Here's how the part is built. I have some questions about the finished solid (model axes, mm). Face numbers are marked on the shaded views. A direction names the side the tool comes from. Give positions to 0.01 mm unless a question says otherwise; leave off trailing zeros. Loops run counter-clockwise (first coordinate to the right, second up) from the corner with the lowest first, then second, coordinate; pieces in that order, holes last. Notation, with made-up numbers: (7.25, 47) - (27.25, 47) arc R25 ccw to (27.25, 85) - close; hole circle Ø1 at (84.25, -5.75). An arc over 180 degrees is marked (long way). Use a Markdown table: item, result.
Solid Edge part; units mm, degrees
sketch "Sketch1" plane through (0, 0, 0) normal (0, 0, 1) x (1, 0, 0)
  circle A0 centre (-61.7143, 32.036) radius 10
extrude "Protrusion1" add sketch "Sketch1" along normal blind 35
sketch "Sketch2" plane through (-61.7143, 32.036, 35) normal (0, 0, 1) x (1, 0, 0)
  line L0 (-35, -15) -> (35, -15)
  line L1 (35, -15) -> (35, 105)
  line L2 (35, 105) -> (-35, 105)
  line L3 (-35, 105) -> (-35, -15)
  dimension "D1" = 35
  dimension "D2" = 35
extrude "ExtrudedProtrusion_2" add sketch "Sketch2" along normal blind 10
sketch "Sketch3" plane through (-61.7143, 32.036, 0) normal (0, 0, -1) x (1, 0, 0)
  circle A0 centre (0, 0) radius 4
extrude "Cutout1" cut sketch "Sketch3" against normal through all
properties material "Aluminum, 6061-T6"
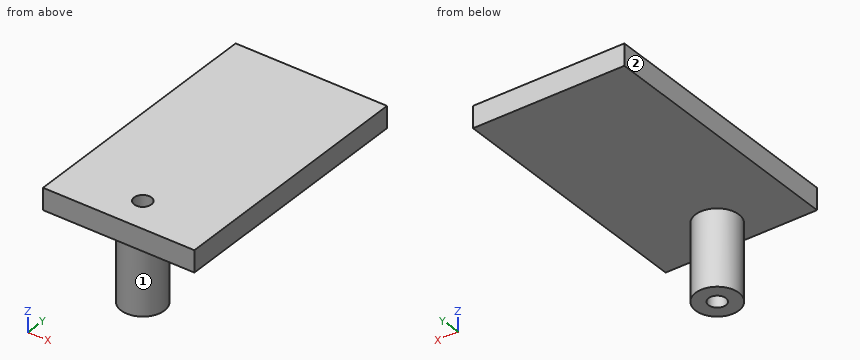
(1) If I drill on line 1 (Z direction, x = -52, y = 106.5); line 2 (Y direction, x = -59.5, z = 30); line 3 (Y direction, x = -60, z = 4.5), over which ranges is the centre line in solid material (lowest first)?
A:
| item | result |
|---|---|
| line 1 | 35 to 45 |
| line 2 | 22.28 to 28.7, 35.37 to 41.79 |
| line 3 | 22.18 to 28.42, 35.65 to 41.89 |
(2) Will these pins go through, and if not, where does the flat tip stop? pin 1 (21 mm diameter, centred on x = -70.5, y = 65, fed in from -Z); pin 2 (3 mm diameter, centred on x = -54, z = 15.5, fed in from +Y).
A:
| item | result |
|---|---|
| pin 1 | z = 35 |
| pin 2 | y = 39.87 |
(3) On a 3-axis mill with a long thin cutter (end or side, diameter ignored), from which of +Z, -Z, +X, -X, +Y, -Y can I reach the whole of each face in a straight line? I mean the marked faces 1 and 2. Say none if no direction works.
A:
| item | result |
|---|---|
| face 1 | -Z |
| face 2 | +Z, -Z, -X, +Y, -Y |
(4) Suppose I cut it at A-A on x = -62. Write out the boundary of the cut face in (y, z).
A:
| item | result |
|---|---|
| outline | (17.04, 35) - (22.04, 35) - (22.04, 0) - (28.05, 0) - (28.05, 45) - (17.04, 45) - close; (36.03, 0) - (42.03, 0) - (42.03, 35) - (137.04, 35) - (137.04, 45) - (36.03, 45) - close |
(5) Suppose I cut it at B-B on y = 108.5. Write out the boundary of the cut face in (x, z).
A:
| item | result |
|---|---|
| outline | (-96.71, 35) - (-26.71, 35) - (-26.71, 45) - (-96.71, 45) - close |
(6) Suppose I cut it at D-D on x = -87.5. Write out the boundary of the cut face in (y, z), plus the area to 3 significant figures.
A:
| item | result |
|---|---|
| outline | (17.04, 35) - (137.04, 35) - (137.04, 45) - (17.04, 45) - close |
| area | 1,200 mm2 |
(7) Suppose I cut it at C-C on z = 11.5. Write out the boundary of the cut face in (x, y).
A:
| item | result |
|---|---|
| outline | circle Ø20 at (-61.71, 32.04); hole circle Ø8 at (-61.71, 32.04) |
